Geometry check sheet. Reference: the model listing, model coordinates, mm. Give positions to 0.01 mm unless a question says otherwise; leave off trailing zeros. Loops run counter-clockwise (first coordinate to the right, second up) from the corner with the lowest first, then second, coordinate; pieces in that order, holes last.
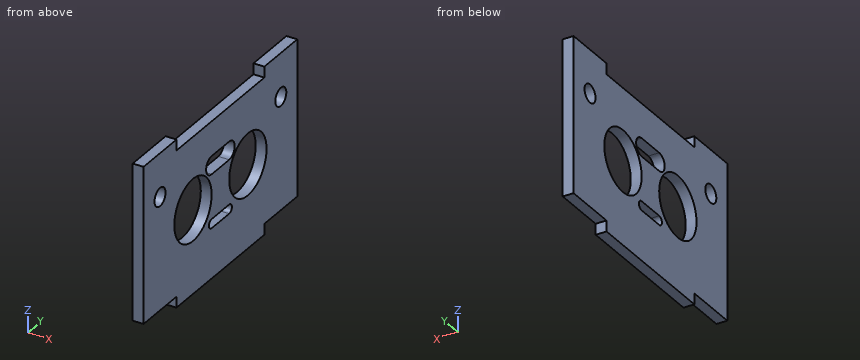
```python
from build123d import *

# Parameters (mm, degrees)
PAD002_DEPTH    = 3
SKETCH008_R     = 8.5
POCKET005_DEPTH = 3.001
SKETCH009_R     = 2.5
POCKET006_DEPTH = 3.001


with BuildPart() as part:
    # Sketch007 → Pad002 (new body)
    with BuildSketch(Plane.YZ):
        Polygon((-35, 43), (-20, 43), (-20, 40), (20, 40), (20, 43), (35, 43), (35, 0), (20, 0), (20, -3), (-20, -3), (-20, 0), (-35, 0), align=None)
    extrude(amount=PAD002_DEPTH)

    # Sketch008 → Pocket005 (cut, through all)
    with BuildSketch(Plane.YZ.offset(3)):
        with Locations((-12.5, 20)):
            Circle(SKETCH008_R)
        with Locations((12.5, 20)):
            Circle(SKETCH008_R)
        with BuildLine():
            Line((-4, 30.5), (4, 30.5))
            ThreePointArc((4, 25.5), (6.5, 28), (4, 30.5))
            Line((-4, 25.5), (4, 25.5))
            ThreePointArc((-4, 30.5), (-6.5, 28), (-4, 25.5))
        make_face()
        with BuildLine():
            Line((-4, 13.25), (4, 13.25))
            ThreePointArc((4, 10.75), (5.25, 12), (4, 13.25))
            Line((-4, 10.75), (4, 10.75))
            ThreePointArc((-4, 13.25), (-5.25, 12), (-4, 10.75))
        make_face()
    extrude(amount=-POCKET005_DEPTH, mode=Mode.SUBTRACT)

    # Sketch009 → Pocket006 (cut, through all)
    with BuildSketch(Plane.YZ.offset(3)):
        with Locations((-27.5, 31)):
            Circle(SKETCH009_R)
        with Locations((27.5, 31)):
            Circle(SKETCH009_R)
    extrude(amount=-POCKET006_DEPTH, mode=Mode.SUBTRACT)


solid = part.part
```
1) Scan lines: line 1 along Z through (x, y) = (1.05, 1.5); line 2 along Z through (x, y) = (1.45, 5.5); line 3 along Y through (x, z) = (2.8, 27). Record each from-to range of solid material in increasing order.
2) Depth check by flat-ended pin: P1, Ø1.5, axis at x = 2, z = -1, coming from the -Y side; P2, Ø1.5, axis at x = 1, y = 6.5, coming from the +Z side; P3, Ø1.5, axis at x = 0.5, y = 24, coming from the -Z side. Enter the tip coordinate at first touch or a pass-through.
3) Sectioned sample at C-C on x = 2.5. Enter the section's corners in (y, z).
4) Sectioned sample at D-D on y = 12.5. Enter the section's corners in (x, z).
5) Sectioned sample at B-B on z = 24.5. Enter the section's corners in (x, y), plus the area to 3 significant figures.
6) Sectioned sample at A-A on y = -27.5. Enter the section's corners in (x, z), plus the area to 3 significant figures.
Determined:
1. line 1: z = -3 to 10.75, 13.25 to 25.5, 30.5 to 40
1. line 2: z = -3 to 15.18, 24.82 to 26, 30 to 40
1. line 3: y = -35 to -17.32, -7.68 to -6.29, 6.29 to 7.68, 17.32 to 35
2. P1: stops at y = -20
2. P2: stops at z = 40
2. P3: stops at z = 0
3. outline: (-35, 0) - (-20, 0) - (-20, -3) - (20, -3) - (20, 0) - (35, 0) - (35, 43) - (20, 43) - (20, 40) - (-20, 40) - (-20, 43) - (-35, 43) - close; hole circle Ø5 at (-27.5, 31); hole circle Ø17 at (-12.5, 20); hole (-4, 10.75) - (4, 10.75) arc R1.25 ccw to (4, 13.25) - (-4, 13.25) arc R1.25 ccw to start; hole (-4, 25.5) - (4, 25.5) arc R2.5 ccw to (4, 30.5) - (-4, 30.5) arc R2.5 ccw to start; hole circle Ø17 at (12.5, 20); hole circle Ø5 at (27.5, 31)
4. outline: (0, -3) - (3, -3) - (3, 11.5) - (0, 11.5) - close; (0, 28.5) - (3, 28.5) - (3, 40) - (0, 40) - close
5. outline: (0, -35) - (3, -35) - (3, -19.71) - (0, -19.71) - close; (0, -5.29) - (3, -5.29) - (3, 5.29) - (0, 5.29) - close; (0, 19.71) - (3, 19.71) - (3, 35) - (0, 35) - close
5. area: 123 mm2
6. outline: (0, 0) - (3, 0) - (3, 28.5) - (0, 28.5) - close; (0, 33.5) - (3, 33.5) - (3, 43) - (0, 43) - close
6. area: 114 mm2
